Verification items for this drawing (mm, ordinates from the low corner). Round coordinates to 2 decimals unless told otherwise and drop trailing zeros. Write each loop counter-clockwise with the first axis right and the second up, starting at its lowest first coordinate (ties: lowest second). Pieces come first, ordered by that corner, then holes. Notation, with made-up numbers: (-21, 27) -> (37, 27) arc R25 cw to (37, 57) -> close; hole circle Ø4 at (51, 59). An arc over 180 degrees is marked (long way). One line per item, written item: value.
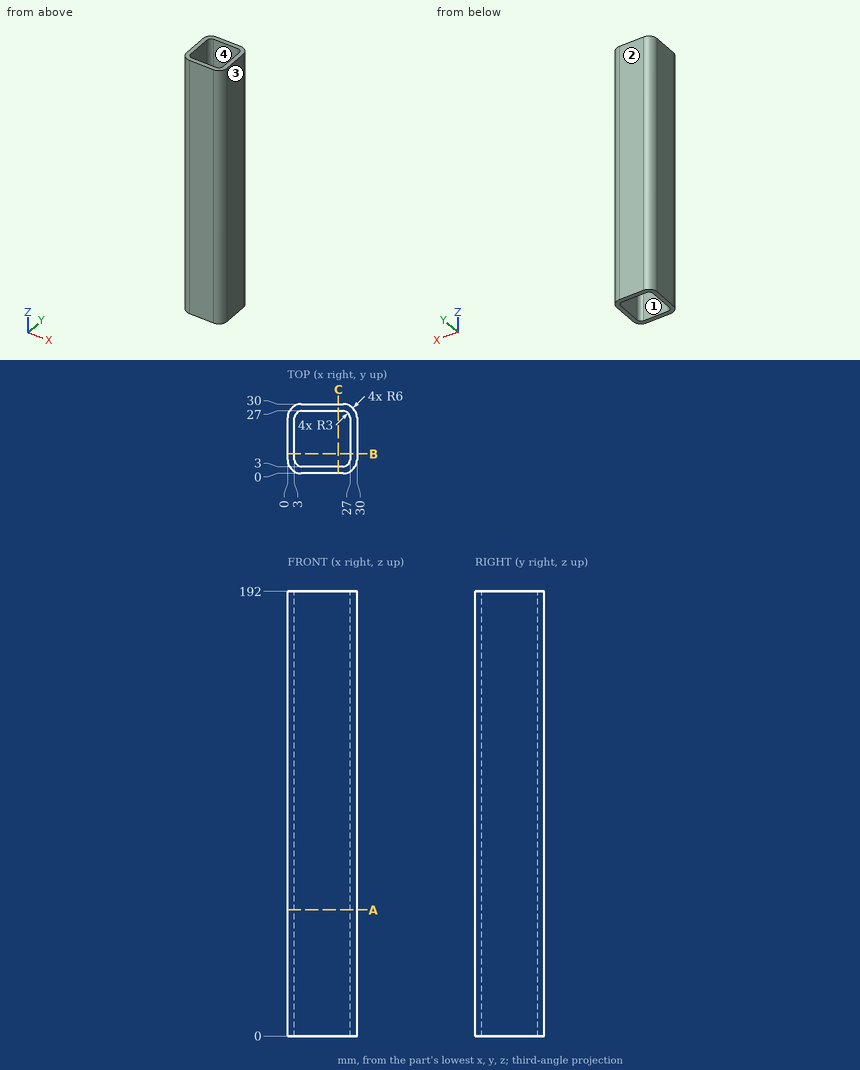
Item 1: Sectioned sample at B-B (y = 8.5). Enter the section's corners in (x, z), then the cut area to 3 significant figures.
Result set:
outline: (0, 0) -> (3, 0) -> (3, 192) -> (0, 192) -> close; (27, 0) -> (30, 0) -> (30, 192) -> (27, 192) -> close
area: 1,150 mm^2
Item 2: Release check for a two-part mould opening along X. For the marked faces 1, 2, 3 and 4 record: pulls with the +X half, pulls with the -X half, needs draft (parallel to the pull), parting line crosses it, or undercut.
Result set:
face 1: undercut
face 2: needs draft
face 3: pulls with the +X half
face 4: undercut
Item 3: Material ranges on line 1 along Y through (x, z) = (14.25, 150.5); line 2 along Y through (x, z) = (3.25, 152), recorded low to high.
Result set:
line 1: 0 to 3, 27 to 30
line 2: 0.67 to 4.8, 25.2 to 29.33
Item 4: Sectioned sample at A-A (z = 54.5). Enter the section's corners in (x, y), then the cut area to 3 significant figures.
Result set:
outline: (0, 6) arc R6 ccw to (6, 0) -> (24, 0) arc R6 ccw to (30, 6) -> (30, 24) arc R6 ccw to (24, 30) -> (6, 30) arc R6 ccw to (0, 24) -> close; hole (3, 6) arc R3 ccw to (6, 3) -> (24, 3) arc R3 ccw to (27, 6) -> (27, 24) arc R3 ccw to (24, 27) -> (6, 27) arc R3 ccw to (3, 24) -> close
area: 301 mm^2
